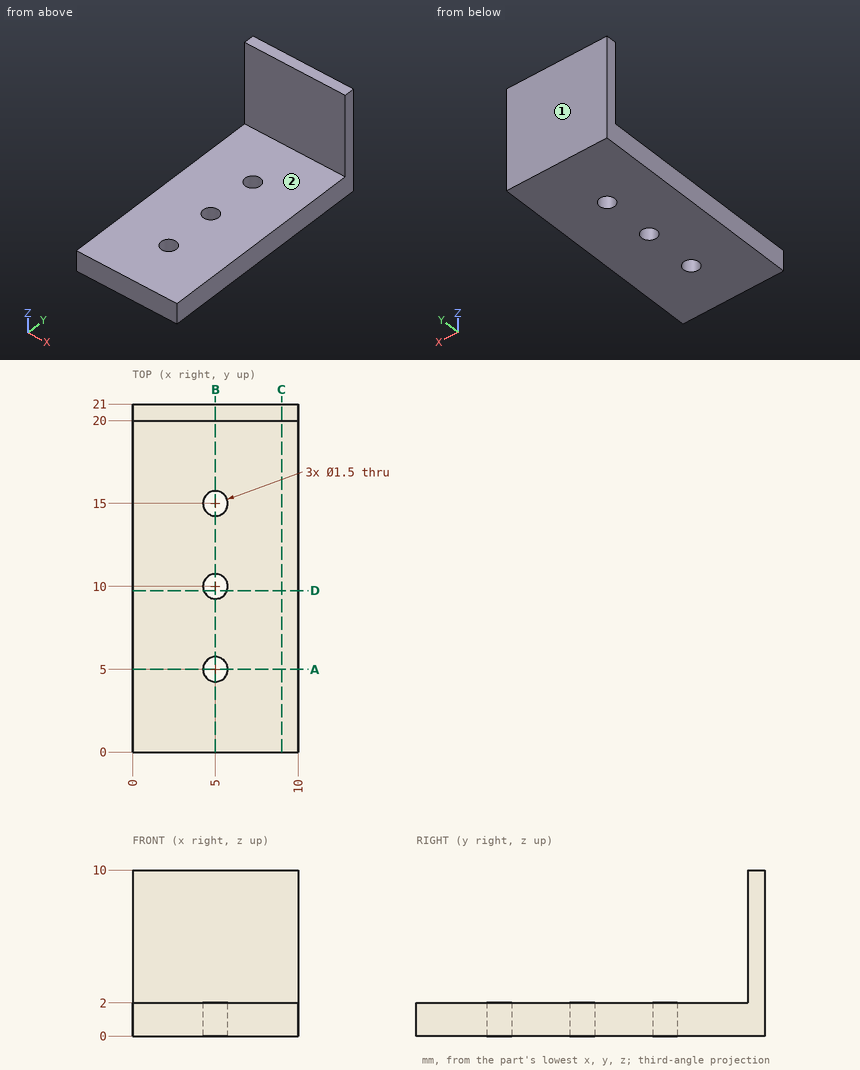
Answer from the drawing. Dimensions are ordinates in mm from the lowest x, y and z of the part. A direction names the side the tool comes from. Give positions to 0.01 mm unless a question says otherwise; leave off trailing zeros. Order: outer loops, then holes, each group sorted by start corner. A loop starts at its lowest first (then second) coordinate and runs counter-clockwise, first axis right, second up. Notation, with made-up numbers: (-7, 87) - (19, 87) arc R17 ccw to (19, 99) - close; hole circle Ø10 at (17.5, 55). An arc over 180 degrees is marked (long way). Use one line per item in the form item = value.
1) Consider probe 1 along Y at (x, z) = (5, 0.9); probe 2 along Y at (x, z) = (1.25, 9.25); probe 3 along Z at (x, y) = (3.75, 4). Determine where each line is inside the solid, lowest interval first. Write a range as [from, to].
Verdict:
probe_1 = [0, 4.25], [5.75, 9.25], [10.75, 14.25], [15.75, 21]
probe_2 = [20, 21]
probe_3 = [0, 2]
2) Find section A-A on y = 5. Determine the outline of the cut face in (x, z), and give its area (3 significant figures).
Verdict:
outline = (0, 0) - (4.25, 0) - (4.25, 2) - (0, 2) - close; (5.75, 0) - (10, 0) - (10, 2) - (5.75, 2) - close
area = 17.0 mm^2
3) Each of these flat-tipped pins is pushed along its axis until it touches: pin 1 (4 mm diameter, centred on x = 7.5, z = 3.5, fed in from -Y); pin 2 (1 mm diameter, centred on x = 5, y = 15, fed in from -Z); pin 3 (1 mm diameter, centred on x = 4, z = 8, fed in from -Y); pin 4 (3 mm diameter, centred on x = 4.5, y = 5, fed in from +Z). Where does it stop, or does it pass through?
Verdict:
pin_1 = 0
pin_2 = through
pin_3 = 20
pin_4 = 2
4) Find section B-B on x = 5. Determine the outline of the cut face in (y, z).
Verdict:
outline = (0, 0) - (4.25, 0) - (4.25, 2) - (0, 2) - close; (5.75, 0) - (9.25, 0) - (9.25, 2) - (5.75, 2) - close; (10.75, 0) - (14.25, 0) - (14.25, 2) - (10.75, 2) - close; (15.75, 0) - (21, 0) - (21, 10) - (20, 10) - (20, 2) - (15.75, 2) - close
5) For the marked faces 1 and 2, determine the directions among +Z, -Z, +X, -X, +Y, -Y from which every point of the face is accessible in a straight line to the end or side of a thin tool.
Verdict:
face_1 = +Z, -Z, +X, -X, +Y
face_2 = +Z, +X, -X, -Y
6) Find section D-D on y = 9.75. Determine the outline of the cut face in (x, z).
Verdict:
outline = (0, 0) - (4.29, 0) - (4.29, 2) - (0, 2) - close; (5.71, 0) - (10, 0) - (10, 2) - (5.71, 2) - close
7) Find section C-C on x = 9. Determine the outline of the cut face in (y, z), and give its area (3 significant figures).
Verdict:
outline = (0, 0) - (21, 0) - (21, 10) - (20, 10) - (20, 2) - (0, 2) - close
area = 50.0 mm^2
